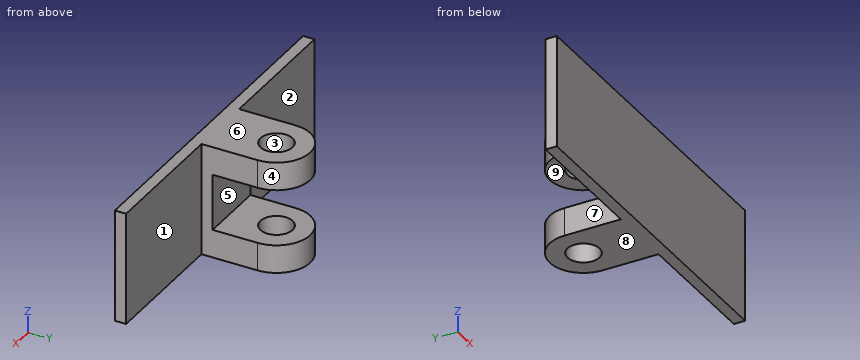
Autodesk Inventor part; units mm, degrees
ref_plane "YZ Plane" through (0, 0, 0) normal (1, 0, 0) x (0, 1, 0)
ref_plane "XZ Plane" through (0, 0, 0) normal (0, 1, 0) x (-1, 0, 0)
ref_plane "XY Plane" through (0, 0, 0) normal (0, 0, 1) x (1, 0, 0)
sketch "Sketch1" plane through (0, 0, 0) normal (0, 1, 0) x (-1, 0, 0)
  line L0 (0, 0) -> (30, 0)
  line L1 (30, 0) -> (30, -10)
  line L2 (30, -10) -> (0, -10)
  line L3 (0, -10) -> (0, 0)
  dimension "d0" = 10
  dimension "d1" = 30
extrude "Extrusion1" add sketch "Sketch1" along normal blind 1
sketch "Sketch2" plane through (0, 1, 0) normal (0, 1, 0) x (1, 0, 0)
  line L0 (-30, 10) -> (-30, 0)
  line L1 (-30, 5) -> (-15, 5)
  line L2 (-15, 5) -> (-15, 2.5)
  line L3 (-15, 2.5) -> (-18, 2.5)
  line L4 (-18, 2.5) -> (-12, 2.5)
  line L5 (-12, 2.5) -> (-12, 0)
  line L6 (-12, 0) -> (-18, 0)
  line L7 (-18, 0) -> (-18, 2.5)
  line L8 (-15, 5) -> (-15, 7.5)
  line L9 (-15, 7.5) -> (-18, 7.5)
  line L10 (-18, 7.5) -> (-12, 7.5)
  line L11 (-12, 7.5) -> (-12, 10)
  line L12 (-12, 10) -> (-18, 10)
  line L13 (-18, 10) -> (-18, 7.5)
  point P0 (0, 0)
  dimension "d4" = 15
  dimension "d5" = 2.5
  dimension "d20" = 3
  dimension "d21" = 2.5
  dimension "d22" = 6
  dimension "d23" = 2.5
  dimension "d24" = 3
  dimension "d25" = 2.5
  dimension "d26" = 6
extrude "Extrusion2" add sketch "Sketch2" along normal blind 8
sketch "Sketch4" plane through (-30, 0, 0) normal (0, 0, 1) x (1, 0, 0)
  line L0 (12, 9) -> (18, 9)
  line L1 (15, 9) -> (15, 6)
  circle A0 centre (15, 6) radius 3
  circle A1 centre (15, 6) radius 1.425
  line L2 (18, 1) -> (18, 9)
  line L3 (12, 9) -> (18, 9)
  line L4 (18, 9) -> (18, 3)
  line L5 (18, 3) -> (12, 3)
  line L6 (12, 3) -> (12, 9)
  point P0 (30, 0)
  point P1 (12, 6)
  point P2 (18, 6)
  dimension "d27" = 3
  dimension "d28" = 2.85
extrude "Extrusion4" cut sketch "Sketch4" against normal through all contours L0 A0 L6 | A1 | L0 L2 A0
sketch "Sketch5" plane through (0, 1, 0) normal (0, 1, 0) x (1, 0, 0)
  line L0 (-18, 2.5) -> (-18, 0)
  line L1 (-12, 7.5) -> (-18, 7.5)
  line L2 (-18, 2.5) -> (-12, 2.5)
  line L3 (-12, 2.5) -> (-12, 7.5)
  line L4 (-12, 7.5) -> (-18, 7.5)
  line L5 (-18, 7.5) -> (-18, 2.5)
  point P0 (0, 0)
extrude "Extrusion5" add sketch "Sketch5" along normal blind 1
properties part number "FingerTip"
The listing builds one solid part. Answer for the finished solid, in the listing's coordinates (mm). Face numbers are marked on the shaded views. A direction names the side the tool comes from. Give positions to 0.01 mm unless a question says otherwise; leave off trailing zeros. Write each loop counter-clockwise with the first axis right and the second up, starting at its lowest first coordinate (ties: lowest second). Pieces come first, ordered by that corner, then holes. Notation, with made-up numbers: (51.25, 9) -> (100.25, 9) arc R17 cw to (100.25, 40) -> close; hole circle Ø1 at (-13.5, -38.75). An arc over 180 degrees is marked (long way). Use one line per item in the form item = value.
1) For a pull along Z with two mould halves and no side action, classify the marked faces 6, 7, 8 and 9 as +Z half, -Z half, draft (parallel to the pull), parting line (faces both ways), or undercut.
Result:
face_6 = +Z half
face_7 = draft
face_8 = -Z half
face_9 = undercut
2) Section C-C on z = -8.5 is taken. Write down the section's boundary in (x, y) (3 decimals), plus the area to 3 significant figures.
Result:
outline = (-30, 0) -> (0, 0) -> (0, 1) -> (-12, 1) -> (-12, 6) arc R3 ccw to (-18, 6) -> (-18, 1) -> (-30, 1) -> close; hole circle Ø2.85 at (-15, 6)
area = 67.8 mm²
3) Section A-A on x = -15 is taken. Write down the section's boundary in (y, z) (3 decimals).
Result:
outline = (0, -10) -> (4.575, -10) -> (4.575, -7.5) -> (2, -7.5) -> (2, -2.5) -> (4.575, -2.5) -> (4.575, 0) -> (0, 0) -> close; (7.425, -10) -> (9, -10) -> (9, -7.5) -> (7.425, -7.5) -> close; (7.425, -2.5) -> (9, -2.5) -> (9, 0) -> (7.425, 0) -> close
4) Section B-B on y = 4 is taken. Write down the section's boundary in (x, z), plus the area to 3 significant figures.
Result:
outline = (-18, -10) -> (-12, -10) -> (-12, -7.5) -> (-18, -7.5) -> close; (-18, -2.5) -> (-12, -2.5) -> (-12, 0) -> (-18, 0) -> close
area = 30.0 mm²
5) A tool of negligible diameter and unlimited length cuts with its end or side. For the marked faces 1, 2, 3, 4 and 5, from which of +Z, -Z, +X, -X, +Y, -Y can it reach the whole face along a straight path? Write none if from no direction.
Result:
face_1 = +Z, -Z, +X, +Y
face_2 = +Z, -Z, -X, +Y
face_3 = +Z, -Z
face_4 = +Z, -Z, +Y
face_5 = +X, -X, +Y
6) Each of these flat-tipped pins is pushed along its axis until it touches: P1, Ø1.7, axis at x = -15, y = 6, coming from the +Z side; P2, Ø4, axis at y = 5.5, z = -3.5, coming from the -X side. Where does it stop, or does it pass through?
Result:
P1 = through
P2 = -18
7) Section D-D on y = 7 is taken. Write down the section's boundary in (x, z).
Result:
outline = (-17.83, -10) -> (-16.02, -10) -> (-16.02, -7.5) -> (-17.83, -7.5) -> close; (-17.83, -2.5) -> (-16.02, -2.5) -> (-16.02, 0) -> (-17.83, 0) -> close; (-13.98, -10) -> (-12.17, -10) -> (-12.17, -7.5) -> (-13.98, -7.5) -> close; (-13.98, -2.5) -> (-12.17, -2.5) -> (-12.17, 0) -> (-13.98, 0) -> close
8) Straight lines are drawn through the part: probe 1 along Y at (x, z) = (-15, -1.05) (3 decimals); probe 2 along X at (y, z) = (6, -1.7) (3 decimals); probe 3 along Y at (x, z) = (-8.5, -9). For each, find the intervals that lie inside material, in ascending order.
Result:
probe_1 = 0 to 4.575, 7.425 to 9
probe_2 = -18 to -16.425, -13.575 to -12
probe_3 = 0 to 1
